Geometry: final body of the model. Coordinates: model frame, mm. A direction names the side the tool comes from. Give positions to 0.01 mm unless a question says otherwise; leave off trailing zeros. Write each loop counter-clockwise with the first axis right and the second up, starting at its lowest first coordinate (ties: lowest second). Pieces come first, ordered by that corner, then holes. Notation, with made-up numbers: (78.5, 54.5) -> (86.5, 54.5) arc R29 cw to (86.5, 78.5) -> close; hole circle Ø5 at (44, 48). An arc over 180 degrees is marked (long way). Answer in a Markdown table with one row per item. Add a question column.
Item 1: Material intervals for probe 1 along Y at (x, z) = (-128, 7.5); probe 2 along X at (y, z) = (110, 60.5); probe 3 along Y at (x, z) = (-119, 70.5), sorted ascending. Write a range as from..to.
Item 2: Section query B-B on x = -57. Output: boundary loops of the cut face in (y, z).
Item 3: Draft query along Y for faces 1 (the flat face through (-184.976, 106, 40)), 2 (the cylindrical face through (-178.466, 72.535, 41.031)), 3 (the cylindrical face through (-179.864, 71.105, 40.017)). Return one class per face: +Y half, -Y half, draft (parallel to the pull), parting line (faces both ways), or undercut.
Item 4: Section query A-A on z = 27. Output: boundary loops of the cut face in (x, y).
Item 5: Section query C-C on y = 91. Output: boundary loops of the cut face in (x, z), plus the area to 3 significant figures.
Item 6: First-contact query: P1, Ø4, axis at x = -108.5, y = 136, coming from the +Z side. Flat tip, straight axial feed; report the tip coordinate or a pass-through.
Item 7: Access query for faces 4 (the cylindrical face through (-40.09, 141.41, 40.02)), 5 (the cylindrical face through (-38.78, 106.58, 3.71)). Directions: +Z, -Z, +X, -X, +Y, -Y. A direction counts if a zero-diameter tool reaches every point of the face in a straight line with its end or side. Return the directions, or none.
```python
from build123d import *

# Parameters (mm, degrees)
BOSS_EXTRUDE1_DEPTH = 75
BOSS_EXTRUDE2_DEPTH = 2
FILLET1_R           = 6


with BuildPart() as part:
    # Sketch2 → Boss-Extrude1 (new body)
    with BuildSketch(Plane.XY):
        with BuildLine():
            Line((-167.97646099, 146.257283518), (-51.97646099, 146.257283518))
            ThreePointArc((-51.97646099, 146.257283518), (-39.95564571, 141.278098799), (-34.97646099, 129.257283518))
            Line((-34.97646099, 129.257283518), (-34.97646099, 83.257283518))
            ThreePointArc((-34.97646099, 83.257283518), (-39.95564571, 71.236468238), (-51.97646099, 66.257283518))
            Line((-51.97646099, 66.257283518), (-167.97646099, 66.257283518))
            ThreePointArc((-167.97646099, 66.257283518), (-179.99727627, 71.236468238), (-184.97646099, 83.257283518))
            Line((-184.97646099, 83.257283518), (-184.97646099, 129.257283518))
            ThreePointArc((-184.97646099, 129.257283518), (-179.99727627, 141.278098799), (-167.97646099, 146.257283518))
        make_face()
        with BuildLine():
            Line((-167.97646099, 144.257283518), (-51.97646099, 144.257283518))
            ThreePointArc((-51.97646099, 144.257283518), (-41.369859272, 139.863885236), (-36.97646099, 129.257283518))
            Line((-36.97646099, 129.257283518), (-36.97646099, 83.257283518))
            ThreePointArc((-36.97646099, 83.257283518), (-41.369859272, 72.650681801), (-51.97646099, 68.257283518))
            Line((-51.97646099, 68.257283518), (-167.97646099, 68.257283518))
            ThreePointArc((-167.97646099, 68.257283518), (-178.583062708, 72.650681801), (-182.97646099, 83.257283518))
            Line((-182.97646099, 83.257283518), (-182.97646099, 129.257283518))
            ThreePointArc((-182.97646099, 129.257283518), (-178.583062708, 139.863885236), (-167.97646099, 144.257283518))
        make_face(mode=Mode.SUBTRACT)
    extrude(amount=BOSS_EXTRUDE1_DEPTH)

    # Sketch3 → Boss-Extrude2 (add)
    with BuildSketch(Plane(origin=(0, 0, 0), x_dir=(-1, 0, 0), z_dir=(0, 0, -1))):
        with BuildLine():
            Line((34.97646099, 129.257283518), (34.97646099, 83.257283518))
            ThreePointArc((34.97646099, 83.257283518), (39.95564571, 71.236468238), (51.97646099, 66.257283518))
            Line((51.97646099, 66.257283518), (167.97646099, 66.257283518))
            ThreePointArc((167.97646099, 66.257283518), (179.99727627, 71.236468238), (184.97646099, 83.257283518))
            Line((184.97646099, 83.257283518), (184.97646099, 129.257283518))
            ThreePointArc((184.97646099, 129.257283518), (179.99727627, 141.278098799), (167.97646099, 146.257283518))
            Line((167.97646099, 146.257283518), (51.97646099, 146.257283518))
            ThreePointArc((51.97646099, 146.257283518), (39.95564571, 141.278098799), (34.97646099, 129.257283518))
        make_face()
    extrude(amount=-BOSS_EXTRUDE2_DEPTH)

    # Fillet1
    fillet1_edges = [part.edges().sort_by_distance(p)[0] for p in [
        (-184.97646099, 106.257283518, 0),
        (-179.99727627, 141.278098799, 0),
        (-109.97646099, 146.257283518, 0),
        (-39.95564571, 141.278098799, 0),
        (-109.97646099, 144.257283518, 2),
        (-182.97646099, 106.257283518, 2),
        (-178.583062708, 139.863885236, 2),
        (-41.369859272, 139.863885236, 2),
        (-36.97646099, 106.257283518, 2),
        (-41.369859272, 72.650681801, 2),
        (-109.97646099, 68.257283518, 2),
        (-178.583062708, 72.650681801, 2),
        (-34.97646099, 106.257283518, 0),
        (-39.95564571, 71.236468238, 0),
        (-109.97646099, 66.257283518, 0),
        (-179.99727627, 71.236468238, 0),
    ]]
    fillet(fillet1_edges, radius=FILLET1_R)


solid = part.part
```
Findings below:
| question | item | result |
|---|---|---|
| 1 | probe 1 | y = 66.26..68.28, 144.24..146.26 |
| 1 | probe 2 | x = -184.98..-182.98, -36.98..-34.98 |
| 1 | probe 3 | y = 66.26..68.26, 144.26..146.26 |
| 2 | outline | (66.26, 6) arc R6 ccw to (72.26, 0) -> (140.26, 0) arc R6 ccw to (146.26, 6) -> (146.26, 75) -> (144.26, 75) -> (144.26, 8) arc R6 cw to (138.26, 2) -> (74.26, 2) arc R6 cw to (68.26, 8) -> (68.26, 75) -> (66.26, 75) -> close |
| 3 | face 1 | draft |
| 3 | face 2 | undercut |
| 3 | face 3 | -Y half |
| 4 | outline | (-184.98, 83.26) arc R17 ccw to (-167.98, 66.26) -> (-51.98, 66.26) arc R17 ccw to (-34.98, 83.26) -> (-34.98, 129.26) arc R17 ccw to (-51.98, 146.26) -> (-167.98, 146.26) arc R17 ccw to (-184.98, 129.26) -> close; hole (-182.98, 83.26) arc R15 ccw to (-167.98, 68.26) -> (-51.98, 68.26) arc R15 ccw to (-36.98, 83.26) -> (-36.98, 129.26) arc R15 ccw to (-51.98, 144.26) -> (-167.98, 144.26) arc R15 ccw to (-182.98, 129.26) -> close |
| 5 | outline | (-184.98, 6) arc R6 ccw to (-178.98, 0) -> (-40.98, 0) arc R6 ccw to (-34.98, 6) -> (-34.98, 75) -> (-36.98, 75) -> (-36.98, 8) arc R6 cw to (-42.98, 2) -> (-176.98, 2) arc R6 cw to (-182.98, 8) -> (-182.98, 75) -> (-184.98, 75) -> close |
| 5 | area | 592 mm^2 |
| 6 | P1 | stops at z = 2 |
| 7 | face 4 | +Z, -Z, +X, +Y |
| 7 | face 5 | +Z |
